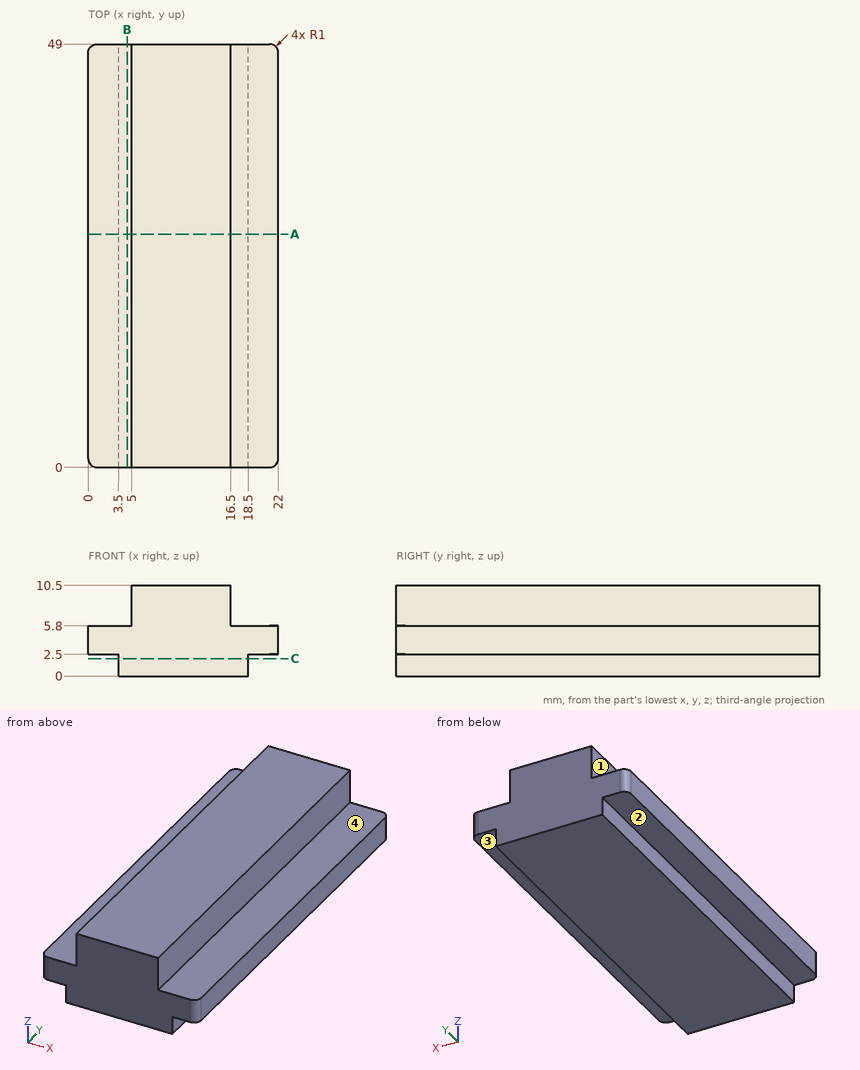
Source: three-view drawing plus pictorial views. Frame: mm from the lowest corner of the part. A direction names the side the tool comes from. Coordinates: 2 decimals unless noted, no trailing zeros. Loops run counter-clockwise (first coordinate to the right, second up) from the corner with the lowest first, then second, coordinate; pieces in that order, holes last. Notation, with made-up numbers: (42, 11.5) -> (56, 11.5) arc R24 cw to (56, 41.5) -> close; hole circle Ø3 at (51.25, 67). An arc over 180 degrees is marked (long way). One line per item, written item: value.
(1) Cut plane B-B (x = 4.5). Output: boundary loops of the cut face in (y, z).
Answer below:
outline: (0, 0) -> (49, 0) -> (49, 5.8) -> (0, 5.8) -> close
(2) Cut plane A-A (y = 27). Output: boundary loops of the cut face in (x, z).
Answer below:
outline: (0, 2.5) -> (3.5, 2.5) -> (3.5, 0) -> (18.5, 0) -> (18.5, 2.5) -> (22, 2.5) -> (22, 5.8) -> (16.5, 5.8) -> (16.5, 10.5) -> (5, 10.5) -> (5, 5.8) -> (0, 5.8) -> close
(3) Pin query (flat end, axial travel): pin 1 Ø3 at (x, y) = (15, 6.5) entering from -Z; pin 2 Ø1.4 at (y, z) = (32.5, 7) entering from -X; pin 3 Ø4 at (y, z) = (18, 9) entering from +X; pin 4 Ø1.8 at (x, y) = (19.5, 25) entering from -Z. Return the tip coordinate at first contact, or that it passes through.
Answer below:
pin 1: stops at z = 0
pin 2: stops at x = 5
pin 3: stops at x = 16.5
pin 4: stops at z = 2.5
(4) Cut plane C-C (z = 2). Output: boundary loops of the cut face in (x, y).
Answer below:
outline: (3.5, 0) -> (18.5, 0) -> (18.5, 49) -> (3.5, 49) -> close
(5) Set-up query: the marked faces 1, 2, 3 and 4. Return all of +Z, -Z, +X, -X, +Y, -Y with unobstructed straight access to the full face (end or side cutting, diameter ignored); none if empty.
Answer below:
face 1: +Z, -X, +Y, -Y
face 2: -Z, -X, +Y, -Y
face 3: -Z, +X, +Y, -Y
face 4: +Z, +X, +Y, -Y
(6) Ray query, line 1 along X through (y, z) = (13.5, 1.75); line 2 along X through (y, z) = (23.5, 8.5); line 3 along Z through (x, y) = (4, 34). Return the intervals inside material, ascending.
Answer below:
line 1: x = 3.5 to 18.5
line 2: x = 5 to 16.5
line 3: z = 0 to 5.8
